```python
from build123d import *

# Parameters (mm, degrees)
SKETCH_1_W             = 80
SKETCH_1_H             = 60
EXTRUDE_1_DEPTH        = 2
SKETCH_3_R             = 2.5
HONEYCOMBCOOLING_DEPTH = 101.019998
SKETCH_4_W             = 20
SKETCH_4_H             = 35
EXTRUDE_2_DEPTH        = 75
SKETCH_5_W             = 18
SKETCH_5_H             = 33
CUT_EXTRUDE_3_DEPTH    = 75
SKETCH_6_W             = 38
SKETCH_6_H             = 31.5
CUT_EXTRUDE_4_DEPTH    = 8
SKETCH_9_W             = 20
SKETCH_9_H             = 25
CUT_EXTRUDE_5_DEPTH    = 10
FILLET_1_R             = 2
FILLET_2_R             = 2


with BuildPart() as part:
    # 草图1 → 凸台-拉伸1 (new body)
    with BuildSketch(Plane.XY):
        with Locations((40, -30)):
            Rectangle(SKETCH_1_W, SKETCH_1_H)
    extrude(amount=EXTRUDE_1_DEPTH)

    # 草图3 → HoneycombCooling (cut, through all)
    with BuildSketch(Plane.XY.offset(2)):
        with Locations((48, -50.784609691)):
            Circle(SKETCH_3_R)
        with Locations((56, -50.784609691)):
            Circle(SKETCH_3_R)
        with Locations((64, -50.784609691)):
            Circle(SKETCH_3_R)
        with Locations((72, -50.784609691)):
            Circle(SKETCH_3_R)
        with Locations((48, -43.856406461)):
            Circle(SKETCH_3_R)
        with Locations((56, -43.856406461)):
            Circle(SKETCH_3_R)
        with Locations((64, -43.856406461)):
            Circle(SKETCH_3_R)
        with Locations((72, -43.856406461)):
            Circle(SKETCH_3_R)
        with Locations((48, -36.92820323)):
            Circle(SKETCH_3_R)
        with Locations((56, -36.92820323)):
            Circle(SKETCH_3_R)
        with Locations((64, -36.92820323)):
            Circle(SKETCH_3_R)
        with Locations((72, -36.92820323)):
            Circle(SKETCH_3_R)
        with Locations((48, -30)):
            Circle(SKETCH_3_R)
        with Locations((56, -30)):
            Circle(SKETCH_3_R)
        with Locations((64, -30)):
            Circle(SKETCH_3_R)
        with Locations((72, -30)):
            Circle(SKETCH_3_R)
        with Locations((48, -23.07179677)):
            Circle(SKETCH_3_R)
        with Locations((56, -23.07179677)):
            Circle(SKETCH_3_R)
        with Locations((64, -23.07179677)):
            Circle(SKETCH_3_R)
        with Locations((72, -23.07179677)):
            Circle(SKETCH_3_R)
        with Locations((48, -16.143593539)):
            Circle(SKETCH_3_R)
        with Locations((56, -16.143593539)):
            Circle(SKETCH_3_R)
        with Locations((64, -16.143593539)):
            Circle(SKETCH_3_R)
        with Locations((72, -16.143593539)):
            Circle(SKETCH_3_R)
        with Locations((48, -9.215390309)):
            Circle(SKETCH_3_R)
        with Locations((56, -9.215390309)):
            Circle(SKETCH_3_R)
        with Locations((64, -9.215390309)):
            Circle(SKETCH_3_R)
        with Locations((72, -9.215390309)):
            Circle(SKETCH_3_R)
    extrude(amount=-HONEYCOMBCOOLING_DEPTH, mode=Mode.SUBTRACT)

    # 草图4 → 凸台-拉伸2 (add)
    with BuildSketch(Plane.XY.offset(2)):
        with Locations((10, -30)):
            Rectangle(SKETCH_4_W, SKETCH_4_H)
    extrude(amount=EXTRUDE_2_DEPTH)

    # 草图5 → 切除-拉伸3 (cut)
    with BuildSketch(Plane.XY.offset(77)):
        with Locations((10, -30)):
            Rectangle(SKETCH_5_W, SKETCH_5_H)
    extrude(amount=-CUT_EXTRUDE_3_DEPTH, mode=Mode.SUBTRACT)

    # 草图6 → 切除-拉伸4 (cut)
    with BuildSketch(Plane(origin=(20, 0, 0), x_dir=(0, 0, -1), z_dir=(1, 0, 0))):
        with Locations((-35, -30)):
            Rectangle(SKETCH_6_W, SKETCH_6_H)
    extrude(amount=-CUT_EXTRUDE_4_DEPTH, mode=Mode.SUBTRACT)

    # 草图9 → 切除-拉伸5 (cut)
    with BuildSketch(Plane(origin=(20, 0, 0), x_dir=(0, 0, -1), z_dir=(1, 0, 0))):
        with Locations((-67, -30)):
            Rectangle(SKETCH_9_W, SKETCH_9_H)
    extrude(amount=-CUT_EXTRUDE_5_DEPTH, mode=Mode.SUBTRACT)

    # 圆角1
    # the kernel refuses this fillet: 2 mm, written as the material it adds along each edge
    with BuildSketch(Plane(origin=(19, -46.5, 77), x_dir=(0, 1, 0), z_dir=(0, 0, -1))) as fillet_1_piece_1_section:
        with BuildLine():
            CenterArc((FILLET_1_R, -FILLET_1_R), FILLET_1_R, 90, 90)
            Line((0, -FILLET_1_R), (0, 0))
            Line((0, 0), (FILLET_1_R, 0))
        make_face()
    fillet_1_piece_1 = extrude(amount=80, mode=Mode.PRIVATE)
    fillet_1_piece_1 = split(fillet_1_piece_1, bisect_by=Plane(origin=(18.871282618, -45.444770831, 54), z_dir=(0, 0, 1)), keep=Keep.TOP, mode=Mode.PRIVATE)
    add(fillet_1_piece_1)
    with BuildSketch(Plane(origin=(19, -46.5, 82), x_dir=(0, 1, 0), z_dir=(0, 0, -1))) as fillet_1_piece_2_section:
        with BuildLine():
            CenterArc((FILLET_1_R, -FILLET_1_R), FILLET_1_R, 90, 90)
            Line((0, -FILLET_1_R), (0, 0))
            Line((0, 0), (FILLET_1_R, 0))
        make_face()
    fillet_1_piece_2 = extrude(amount=80, mode=Mode.PRIVATE)
    fillet_1_piece_2 = split(fillet_1_piece_2, bisect_by=Plane(origin=(18.472438473, -46.20791508, 54), z_dir=(0, 0, -1)), keep=Keep.TOP, mode=Mode.PRIVATE)
    fillet_1_piece_2 = split(fillet_1_piece_2, bisect_by=Plane(origin=(18.472438473, -45.75, 35), z_dir=(0, -1, 0)), keep=Keep.TOP, mode=Mode.PRIVATE)
    add(fillet_1_piece_2)
    with BuildSketch(Plane(origin=(19, -46.5, 82), x_dir=(0, 1, 0), z_dir=(0, 0, -1))) as fillet_1_piece_3_section:
        with BuildLine():
            CenterArc((FILLET_1_R, -FILLET_1_R), FILLET_1_R, 90, 90)
            Line((0, -FILLET_1_R), (0, 0))
            Line((0, 0), (FILLET_1_R, 0))
        make_face()
    fillet_1_piece_3 = extrude(amount=80, mode=Mode.PRIVATE)
    fillet_1_piece_3 = split(fillet_1_piece_3, bisect_by=Plane(origin=(18.871282618, -45.444770831, 16), z_dir=(0, 0, -1)), keep=Keep.TOP, mode=Mode.PRIVATE)
    add(fillet_1_piece_3)
    # the kernel refuses this fillet: 2 mm, written as the material it takes off along each edge
    with BuildSketch(Plane(origin=(0, -47.5, 2), x_dir=(1, 0, 0), z_dir=(0, 0, 1))) as fillet_1_2_piece_1:
        with BuildLine():
            CenterArc((FILLET_1_R, FILLET_1_R), FILLET_1_R, 180, 90)
            Line((0, FILLET_1_R), (0, 0))
            Line((0, 0), (FILLET_1_R, 0))
        make_face()
    extrude(amount=80, mode=Mode.SUBTRACT)
    with BuildSketch(Plane(origin=(0, -12.5, 2), x_dir=(1, 0, 0), z_dir=(0, 0, 1)), Plane(origin=(20, -12.5, 2), x_dir=(0, -1, 0), z_dir=(0, 0, 1))) as fillet_1_2_piece_2:
        with BuildLine():
            CenterArc((FILLET_1_R, -FILLET_1_R), FILLET_1_R, 90, 90)
            Line((0, -FILLET_1_R), (0, 0))
            Line((0, 0), (FILLET_1_R, 0))
        make_face()
    extrude(amount=80, mode=Mode.SUBTRACT)

    # 圆角2
    # the kernel refuses this fillet: 2 mm, written as the material it takes off along each edge
    with BuildSketch(Plane(origin=(20, -47.5, 2), x_dir=(-1, 0, 0), z_dir=(0, 0, 1))) as fillet_2_piece_1:
        with BuildLine():
            CenterArc((FILLET_2_R, -FILLET_2_R), FILLET_2_R, 90, 90)
            Line((0, -FILLET_2_R), (0, 0))
            Line((0, 0), (FILLET_2_R, 0))
        make_face()
    extrude(amount=80, mode=Mode.SUBTRACT)


solid = part.part
```
Build history of the part. All positions in model axes, mm. A direction names the side the tool comes from. Coordinates: 2 decimals unless noted, no trailing zeros. Order: outer loops, then holes, each group sorted by start corner. A loop starts at its lowest first (then second) coordinate and runs counter-clockwise, first axis right, second up.
Item 1: Drill centre lines: L1, parallel to Y at x = 14, z = 42.5; L2, parallel to X at y = -44, z = 71; L3, parallel to X at y = -28, z = 51.5. Where is each one in solid material? Low to high.
Filled in:
L1: y = -47.5 to -46.5, -13.5 to -12.5
L2: x = 0 to 1, 19 to 20
L3: x = 0 to 1
Item 2: Saw through at D-D on x = 11. List the corners of the cut face in (y, z), then the cut area to 3 significant figures.
Filled in:
outline: (-60, 0) - (0, 0) - (0, 2) - (-12.5, 2) - (-12.5, 77) - (-13.5, 77) - (-13.5, 2) - (-46.5, 2) - (-46.5, 77) - (-47.5, 77) - (-47.5, 2) - (-60, 2) - close
area: 270 mm2
Item 3: Drop flat-ended pins along their axis: pin 1 Ø6.5 at (x, y) = (64, -43.86) entering from +Z; pin 2 Ø4 at (x, y) = (56, -16.14) entering from +Z; pin 3 Ø8 at (y, z) = (-39.5, 67.5) entering from +X. Give the stop position or say it passes through.
Filled in:
pin 1: stops at z = 2
pin 2: passes through
pin 3: stops at x = 20
Item 4: Mould opens along X. For faces 4 (the cylindrical face through (65.34, -20.96, 1.01)), 5 (the cylindrical face through (19.43, -13.1, 38.98)), 6 (the cylindrical face through (0.6, -13.07, 38.98)), 7 (the cylindrical face through (66.385, -8.464, 1.014)) say: released by +X, released by -X, zero draft, split by the parting line, or undercut.
Filled in:
face 4: undercut
face 5: released by +X
face 6: released by -X
face 7: undercut
Item 5: Tool access for faces 1 (the cylindrical face through (66.385, -15.393, 1.014)), 2 (the flat face through (19, -29, 15)), 3 (the flat face through (10, -47.5, 39)): list every direction of +Z, -Z, +X, -X, +Y, -Y with a clear straight run to the whole face (end or side of a thin tool).
Filled in:
face 1: +Z, -Z
face 2: +Z
face 3: +Z, +X, -X, -Y
Item 6: Saw through at A-A on y = -30. State how many separate pieces and enclosed holes the cut face has, then the cut area to 3 significant figures.
Filled in:
separate pieces: 6
enclosed holes: 0
area: 212 mm2
Item 7: Saw through at C-C on z = 50. List the corners of the cut face in (x, y), then the cut area to 3 significant figures.
Filled in:
outline: (0, -45.5) arc R2 ccw to (2, -47.5) - (18, -47.5) arc R2 ccw to (19.98, -45.75) - (18.56, -45.75) arc R2 cw to (17, -46.5) - (1, -46.5) - (1, -13.5) - (19, -13.5) - (19, -14.25) - (19.98, -14.25) arc R2 ccw to (18, -12.5) - (2, -12.5) arc R2 ccw to (0, -14.5) - close
area: 71.8 mm2
